Read the model definition and answer for the solid it produces. Units are mm, in the model's axes. A direction names the side the tool comes from. Round coordinates to 2 decimals unless told otherwise and drop trailing zeros. Loops run counter-clockwise (first coordinate to the right, second up) from the corner with the lowest first, then second, coordinate; pieces in that order, holes last. Notation, with made-up numbers: (-19, 68) - (16, 68) arc R30 ccw to (16, 96) - close; hole circle Ø5 at (52, -16.5). An arc over 180 degrees is marked (long way). Use CSV: the item, a comma, the result in double quotes. Start each with the question number.
1. Find section B-B (y = 3). Give the vertices of the cut face in (x, z), and give its area (3 significant figures).
2. A tool of negligible diameter and unlimited length cuts with its end or side. For faces 5 (the flat face through (0, 6, 6)), 6 (the flat face through (9, 6, 6)), from which of +Z, -Z, +X, -X, +Y, -Y can it reach the whole face along a straight path? Write none if from no direction.
3. Find section A-A (x = 3). Give the vertices of the cut face in (y, z).
4. Consider line 1 along Y through (x, z) = (3.35, 9); line 2 along Y through (x, z) = (9, 2.15). Determine where each line is inside the solid, lowest interval first.
5. Determine the mould class of faces 1 (the flat face through (5, 0, 5)), 2 (the flat face through (6, 6, 9)), 3 (the flat face through (5, 12, 5)), 4 (the cylindrical face through (2.958, 2.483, 10.247)) for opening direction Y: +Y half, -Y half, draft (parallel to the pull), parting line (faces both ways), or undercut.
6. Find section D-D (x = 9). Give the vertices of the cut face in (y, z), and give its area (3 significant figures).
7. Given pin 1 Ø1 at (y, z) = (5, 10) entering from +X; pin 2 Ø3 at (x, y) = (10, 5.5) entering from +Z, each flat-ended and moving along its own axis, determine where each tip first touches the part or whether it passes through.
8. Find section C-C (z = 3). Give the vertices of the cut face in (x, y), and give its area (3 significant figures).
Autodesk Inventor part; units mm, degrees
ref_plane "YZ Plane" through (0, 0, 0) normal (1, 0, 0) x (0, 1, 0)
ref_plane "XZ Plane" through (0, 0, 0) normal (0, 1, 0) x (-1, 0, 0)
ref_plane "XY Plane" through (0, 0, 0) normal (0, 0, 1) x (1, 0, 0)
sketch "스케치1" plane through (0, 0, 0) normal (0, 0, 1) x (1, 0, 0)
  line L0 (0, 0) -> (12, 0)
  line L1 (12, 0) -> (12, 12)
  line L2 (12, 12) -> (0, 12)
  line L3 (0, 12) -> (0, 0)
  dimension "d0" = 12
  dimension "d1" = 12
extrude "돌출1" add sketch "스케치1" along normal blind 6
sketch "스케치2" plane through (0, 0, 6) normal (0, 0, 1) x (1, 0, 0)
  line L0 (12, 12) -> (0, 12)
  line L1 (0, 0) -> (6, 0)
  line L2 (6, 0) -> (6, 12)
  line L3 (6, 12) -> (0, 12)
  line L4 (0, 12) -> (0, 0)
extrude "돌출2" add sketch "스케치2" along normal blind 6
sketch "스케치3" plane through (0, 0, 0) normal (0, -1, 0) x (1, 0, 0)
  line L0 (12, 6) -> (6, 6)
  line L1 (6, 6) -> (0, 6)
  line L2 (0, 6) -> (0, 0)
  line L3 (0, 0) -> (6, 0)
  line L4 (6, 0) -> (6, 6)
  circle A0 centre (3, 3) radius 1.35
  dimension "d6" = 2.7
extrude "돌출3" cut sketch "스케치3" against normal up to next contours A0
sketch "스케치4" plane through (0, 0, 0) normal (-1, 0, 0) x (0, 0, 1)
  line L0 (0, 0) -> (12, 0)
  line L1 (12, 0) -> (6, 0)
  line L2 (6, 0) -> (6, 6)
  line L3 (6, 6) -> (12, 6)
  line L4 (12, 6) -> (12, 0)
  circle A0 centre (9, 3) radius 1.35
  dimension "d9" = 2.7
extrude "돌출4" cut sketch "스케치4" against normal up to next contours A0
sketch "스케치5" plane through (0, 0, 6) normal (0, 0, 1) x (1, 0, 0)
  line L0 (12, 0) -> (12, 12)
  line L1 (12, 12) -> (6, 12)
  line L2 (6, 12) -> (6, 6)
  line L3 (6, 6) -> (12, 6)
  line L4 (12, 6) -> (12, 12)
  circle A0 centre (9, 9) radius 1.35
  point P0 (0, 0)
  dimension "d12" = 2.7
extrude "돌출5" cut sketch "스케치5" against normal up to next contours A0
properties part number "부품81"
Filled sheet:
1,outline,"(0, 0) - (12, 0) - (12, 6) - (6, 6) - (6, 7.65) - (0, 7.65) - close; (0, 10.35) - (6, 10.35) - (6, 12) - (0, 12) - close; hole circle Ø2.7 at (3, 3)"
1,area,"86.1 mm²"
2,face 5,"+Z, -Z, -X, +Y, -Y"
2,face 6,"+Z, +X, +Y, -Y"
3,outline,"(0, 0) - (12, 0) - (12, 1.65) - (0, 1.65) - close; (0, 4.35) - (12, 4.35) - (12, 12) - (0, 12) - close; hole circle Ø2.7 at (3, 9)"
4,line 1,"y = 0 to 1.65, 4.35 to 12"
4,line 2,"y = 0 to 7.65, 10.35 to 12"
5,face 1,"-Y half"
5,face 2,"draft"
5,face 3,"+Y half"
5,face 4,"undercut"
6,outline,"(0, 0) - (7.65, 0) - (7.65, 6) - (0, 6) - close; (10.35, 0) - (12, 0) - (12, 6) - (10.35, 6) - close"
6,area,"55.8 mm²"
7,pin 1,"stops at x = 6"
7,pin 2,"stops at z = 6"
8,outline,"(0, 0) - (1.65, 0) - (1.65, 12) - (0, 12) - close; (4.35, 0) - (12, 0) - (12, 12) - (4.35, 12) - close; hole circle Ø2.7 at (9, 9)"
8,area,"106 mm²"
